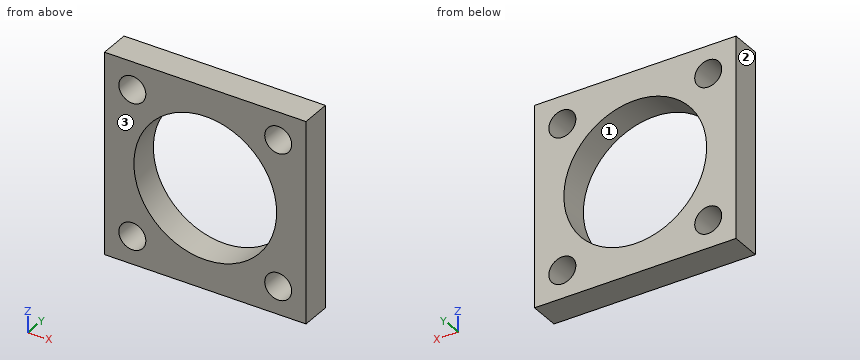
```python
from build123d import *

# Parameters (mm, degrees)
SKETCH2_W            = 25.4
SKETCH2_H            = 25.4
BOSS_EXTRUDE1_DEPTH  = 3.81
SKETCH4_R            = 9
CUT_EXTRUDE1_DEPTH   = 4.81
M3_CLEARANCE_HOLE2_D = 3.4


with BuildPart() as part:
    # Sketch2 → Boss-Extrude1 (new body)
    with BuildSketch(Plane(origin=(0, 0, 0), x_dir=(1, 0, 0), z_dir=(0, 1, 0))):
        Rectangle(SKETCH2_W, SKETCH2_H)
    extrude(amount=BOSS_EXTRUDE1_DEPTH)

    # Sketch4 → Cut-Extrude1 (cut, through all)
    with BuildSketch(Plane(origin=(0, 3.81, 0), x_dir=(1, 0, 0), z_dir=(0, 1, 0))):
        Circle(SKETCH4_R)
    extrude(amount=-CUT_EXTRUDE1_DEPTH, mode=Mode.SUBTRACT)

    # M3 Clearance Hole2 (through all)
    with Locations(Plane(origin=(-9.192388155, 3.81, -9.192388155), x_dir=(0, 0, 1), z_dir=(0, 1, 0))):
        with Locations((0, 0), (18.38477631, 18.38477631), (0, 18.38477631), (18.38477631, 0)):
            Hole(M3_CLEARANCE_HOLE2_D / 2)


solid = part.part
```
For this review, take the finished solid that the model builds, in its own axes (mm). Face numbers are marked on the shaded views. Give positions to 0.01 mm unless a question says otherwise; leave off trailing zeros. Order: outer loops, then holes, each group sorted by start corner. A loop starts at its lowest first (then second) coordinate and runs counter-clockwise, first axis right, second up.
1) The part is to be moulded in two halves that separate along X. For the marked faces 1, 2 and 3, say which applies: released by +X, released by -X, zero draft, split by the parting line, or undercut.
2) Insertion check: pin 1 (2.5 mm diameter, centred on x = -9.19, z = 9.19, fed in from +Y). The pin has a flat end and moves straight along its axis. Give the tip position at first contact, or say it passes through.
3) Take a section at B-B (z = 0). Give the boundary of the cut face in (x, y), then the cut area to 3 significant figures.
4) Wall thickness on line 1 (Z direction, x = 9.25, y = 3.1); line 2 (X direction, y = 3.5, z = 10); line 3 (X direction, y = 1.9, z = -8): over which ranges is each line inside the solid? List them lowest first.
5) Take a section at D-D (x = 8.25). Give the boundary of the cut face in (y, z).
6) Take a section at A-A (x = 0). Give the boundary of the cut face in (y, z), then the cut area to 3 significant figures.
7) Take a section at C-C (x = -10). Give the boundary of the cut face in (y, z), then the cut area to 3 significant figures.
Derived:
1. face 1: undercut
1. face 2: released by -X
1. face 3: zero draft
2. pin 1: passes through
3. outline: (-12.7, 0) - (-9, 0) - (-9, 3.81) - (-12.7, 3.81) - close; (9, 0) - (12.7, 0) - (12.7, 3.81) - (9, 3.81) - close
3. area: 28.2 mm2
4. line 1: z = -12.7 to -10.89, -7.49 to 7.49, 10.89 to 12.7
4. line 2: x = -12.7 to -10.69, -7.7 to 7.7, 10.69 to 12.7
4. line 3: x = -12.7 to -10.4, -7.98 to -4.12, 4.12 to 7.98, 10.4 to 12.7
5. outline: (0, -12.7) - (3.81, -12.7) - (3.81, -10.61) - (0, -10.61) - close; (0, -7.78) - (3.81, -7.78) - (3.81, -3.6) - (0, -3.6) - close; (0, 3.6) - (3.81, 3.6) - (3.81, 7.78) - (0, 7.78) - close; (0, 10.61) - (3.81, 10.61) - (3.81, 12.7) - (0, 12.7) - close
6. outline: (0, -12.7) - (3.81, -12.7) - (3.81, -9) - (0, -9) - close; (0, 9) - (3.81, 9) - (3.81, 12.7) - (0, 12.7) - close
6. area: 28.2 mm2
7. outline: (0, -12.7) - (3.81, -12.7) - (3.81, -10.69) - (0, -10.69) - close; (0, -7.7) - (3.81, -7.7) - (3.81, 7.7) - (0, 7.7) - close; (0, 10.69) - (3.81, 10.69) - (3.81, 12.7) - (0, 12.7) - close
7. area: 74.0 mm2
